```python
from build123d import *

# Parameters (mm, degrees)
SKETCH1_R           = 6.35
BOSS_EXTRUDE1_DEPTH = 3.175
SKETCH2_R           = 6.35
BOSS_EXTRUDE2_DEPTH = 3.175


with BuildPart() as part:
    # Sketch1 → Boss-Extrude1 (new body)
    with BuildSketch(Plane(origin=(0, 0, 0), x_dir=(1, 0, 0), z_dir=(0, 1, 0))):
        Circle(SKETCH1_R)
        Polygon((1.5875, 2.749630657), (-1.5875, 2.749630657), (-3.175, 0), (-1.5875, -2.749630657), (1.5875, -2.749630657), (3.175, 0), align=None, mode=Mode.SUBTRACT)
    extrude(amount=BOSS_EXTRUDE1_DEPTH)

    # Sketch2 → Boss-Extrude2 (add)
    with BuildSketch(Plane(origin=(0, 3.175, 0), x_dir=(1, 0, 0), z_dir=(0, 1, 0))):
        Circle(SKETCH2_R)
        Polygon((1.833087105, 3.175), (-1.833087105, 3.175), (-3.666174209, 0), (-1.833087105, -3.175), (1.833087105, -3.175), (3.666174209, 0), align=None, mode=Mode.SUBTRACT)
    extrude(amount=BOSS_EXTRUDE2_DEPTH)


solid = part.part
```
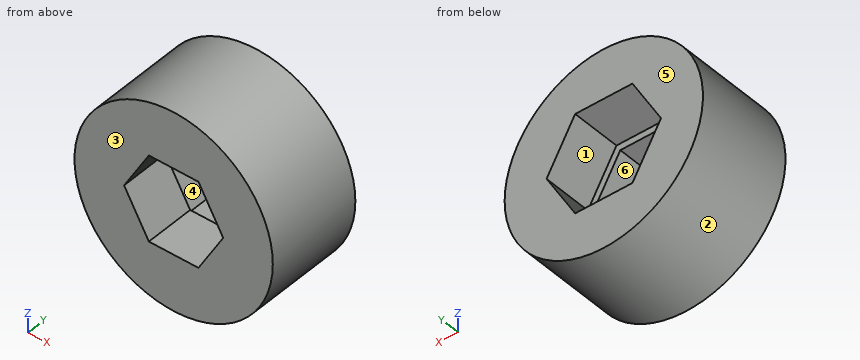
Read the model definition and answer for the solid it produces. Units are mm, in the model's axes. Face numbers are marked on the shaded views. A direction names the side the tool comes from. Coordinates: 2 decimals unless noted, no trailing zeros. Write each loop counter-clockwise with the first axis right and the second up, starting at its lowest first coordinate (ties: lowest second). Pieces come first, ordered by that corner, then holes. Notation, with made-up numbers: (41, 0) -> (81, 0) arc R29 ccw to (81, 22) -> close; hole circle Ø5 at (-21, -10). An arc over 180 degrees is marked (long way). Answer as a JSON object with one key per item and string values.
Q1. Consider line 1 (X direction, y = 5, z = 5.5); line 2 (Z direction, x = 0, y = 5.5) (3 decimals). Determine where each line is inside the solid, lowest interval first. Write a range as [from, to].
The answers:
{"line 1": "x = [-3.17, 3.17]", "line 2": "z = [-6.35, -3.175], [3.175, 6.35]"}
Q2. The part is cut by section C-C on y = 5.75. Give the vertices of the cut face in (x, z) (3 decimals), then the cut area to 3 significant figures.
The answers:
{"outline": "circle Ø12.7 at (0, 0); hole (-3.666, 0) -> (-1.833, -3.175) -> (1.833, -3.175) -> (3.666, 0) -> (1.833, 3.175) -> (-1.833, 3.175) -> close", "area": "91.8 mm2"}
Q3. The part is cut by section A-A on x = 0. Give the vertices of the cut face in (y, z) (3 decimals).
The answers:
{"outline": "(0, -6.35) -> (6.35, -6.35) -> (6.35, -3.175) -> (3.175, -3.175) -> (3.175, -2.75) -> (0, -2.75) -> close; (0, 2.75) -> (3.175, 2.75) -> (3.175, 3.175) -> (6.35, 3.175) -> (6.35, 6.35) -> (0, 6.35) -> close"}
Q4. Flat-ended cylindrical pins translate along their axes: pin 1 Ø2.5 at (x, y) = (-1, 4.5) entering from -Z; pin 2 Ø1.9 at (x, z) = (-0.5, -1) entering from +Y; pin 3 Ø1 at (x, y) = (4.5, 3.5) entering from +Z. Find the tip coordinate at first contact, or state that the pin passes through.
The answers:
{"pin 1": "stops at z = -6.35", "pin 2": "passes through", "pin 3": "stops at z = 4.93"}
Q5. Determine the mould class of the marked faces 1, 2 and 3 for opening direction X: pulls with the +X half, pulls with the -X half, needs draft (parallel to the pull), parting line crosses it, or undercut.
The answers:
{"face 1": "undercut", "face 2": "parting line crosses it", "face 3": "needs draft"}
Q6. The part is cut by section B-B on z = 1. Give the vertices of the cut face in (x, y) (3 decimals), then the cut area to 3 significant figures.
The answers:
{"outline": "(-6.271, 0) -> (-2.598, 0) -> (-2.598, 3.175) -> (-3.089, 3.175) -> (-3.089, 6.35) -> (-6.271, 6.35) -> close; (2.598, 0) -> (6.271, 0) -> (6.271, 6.35) -> (3.089, 6.35) -> (3.089, 3.175) -> (2.598, 3.175) -> close", "area": "43.5 mm2"}
Q7. A tool of negligible diameter and unlimited length cuts with its end or side. For the marked faces 4, 5 and 6, from which of +Z, -Z, +X, -X, +Y, -Y can it reach the whole face along a straight path? Write none if from no direction.
The answers:
{"face 4": "+Y", "face 5": "+Z, -Z, +X, -X, +Y", "face 6": "+Y, -Y"}
